```python
from build123d import *

# Parameters (mm, degrees)
F0_W          = 6.35
F0_H          = 3.175
F1_DEPTH      = 66.04
F2_W          = 6.35
F2_H          = 1.5875
F3_DEPTH      = 3.175
F3_DEPTH_BACK = 6.35
F4_R          = 1.397
F5_DEPTH      = 25.4
F6_R          = 2.54


with BuildPart() as f1:
    # F0 (on Top) → F1 (new body)
    with BuildSketch(Plane.XY):
        with Locations((-3.175, 1.5875)):
            Rectangle(F0_W, F0_H)
    extrude(amount=F1_DEPTH)

    # F2 (on face) → F3 (join, two sides)
    with BuildSketch(Plane(origin=(0, 3.175, 0), x_dir=(-1, 0, 0), z_dir=(0, 1, 0))) as f3_sk:
        with Locations((3.175, 65.24625)):
            Rectangle(F2_W, F2_H)
    extrude(amount=F3_DEPTH)
    extrude(f3_sk.sketch, amount=-F3_DEPTH_BACK)

    # F4 (on face) → F5 (cut)
    with BuildSketch(Plane(origin=(0, 3.175, 0), x_dir=(-1, 0, 0), z_dir=(0, 1, 0))):
        with Locations((3.175, 1.8415)):
            Circle(F4_R)
    extrude(amount=-F5_DEPTH, mode=Mode.SUBTRACT)

    # F6
    f6_edges = [f1.edges().sort_by_distance(p)[0] for p in [
        (-6.35, 1.5875, 0),
        (0, 1.5875, 0),
    ]]
    fillet(f6_edges, radius=F6_R)


solid = f1.part
```
Part model, mm, in its own coordinate system. A direction names the side the tool comes from. Round coordinates to 2 decimals unless told otherwise and drop trailing zeros. Write each loop counter-clockwise with the first axis right and the second up, starting at its lowest first coordinate (ties: lowest second). Pieces come first, ordered by that corner, then holes.
Item 1: Probe L1, parallel to Z at x = -5.5, y = 5.5; L2, parallel to Y at x = -3, z = 5 (3 decimals); L3, parallel to Z at x = -0.75, y = 2.25. List the from-to ranges inside material, lowest first.
Results:
L1: z = 64.45 to 66.04
L2: y = 0 to 3.175
L3: z = 0.74 to 66.04
Item 2: Which spindle directions (+Z, -Z, +X, -X, +Y, -Y) get a long thin tool onto all of the face, cutting with end or side? Do faces 4 (the cylindrical face through (-5.586, 1.61, 0.724)), 5 (the flat face through (-3, 3.175, 32)), 6 (the flat face through (-3, 0, 32)). Say none if no direction does.
Results:
face 4: -Z, -X, +Y, -Y
face 5: -Z, +X, -X, +Y
face 6: -Z, +X, -X, -Y
Item 3: Cut at D-D, the plane y = 5.5. Give the cut face in (x, z), plus the area to 3 significant figures.
Results:
outline: (-6.35, 64.45) - (0, 64.45) - (0, 66.04) - (-6.35, 66.04) - close
area: 10.1 mm2
Item 4: Cut at C-C, the plane z = 15. Give the cut face in (x, y) (3 decimals).
Results:
outline: (-6.35, 0) - (0, 0) - (0, 3.175) - (-6.35, 3.175) - close
Item 5: Two-plate mould, pull along X, no slides. Class faces 1 (the flat face through (-3, 2, 66.04)), 2 (the cylindrical face through (-0.724, 1.61, 0.764)), 3 (the cylindrical face through (-3.82, 1.61, 0.602)): +X half, -X half, draft (parallel to the pull), parting line (faces both ways), or undercut.
Results:
face 1: draft
face 2: +X half
face 3: undercut
Item 6: Drop flat-ended pins along their axis: pin 1 Ø2 at (x, y) = (-3, -1.5) entering from -Z; pin 2 Ø1.5 at (x, z) = (-4.5, 27) entering from -Y; pin 3 Ø3 at (x, z) = (-1.5, 45.5) entering from +Y (3 decimals). Give the stop position or say it passes through.
Results:
pin 1: stops at z = 64.45
pin 2: stops at y = 0
pin 3: stops at y = 3.175
